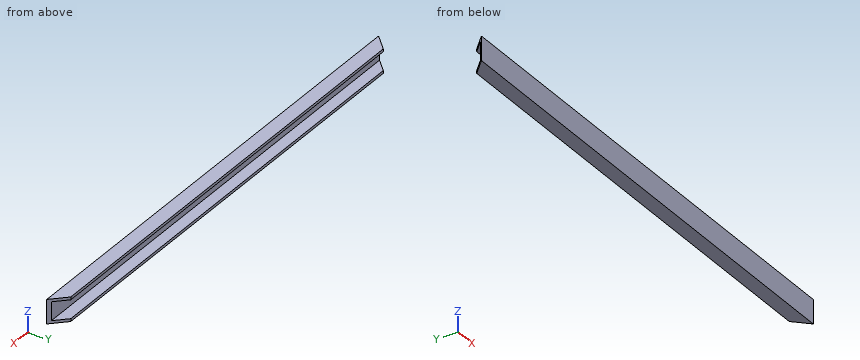
```python
from build123d import *

# Parameters (mm, degrees)
BOSS_EXTRUDE1_DEPTH = 106.2
CUT_EXTRUDE1_DEPTH  = 11.4


with BuildPart() as part:
    # Sketch1 → Boss-Extrude1 (new body, symmetric)
    with BuildSketch(Plane(origin=(0, 0, 0), x_dir=(0, 0, -1), z_dir=(1, 0, 0))):
        Polygon((-4, 5), (-4, 0), (4, 0), (4, 5), (5.2, 5), (5.2, -1.2), (-5.2, -1.2), (-5.2, 5), align=None)
    extrude(amount=BOSS_EXTRUDE1_DEPTH, both=True)

    # Sketch3 → Cut-Extrude1 (cut, through all)
    with BuildSketch(Plane.XY.offset(5.2)):
        Polygon((-106.2, 5), (-106.2, -1.2), (-100, 5), align=None)
        Polygon((106.2, 5), (106.2, -1.2), (100, 5), align=None)
    extrude(amount=-CUT_EXTRUDE1_DEPTH, mode=Mode.SUBTRACT)


solid = part.part
```
Here's how the part is built. I have some questions about the finished solid (model axes, mm). Round coordinates to 2 decimals unless told otherwise and drop trailing zeros. Order: outer loops, then holes, each group sorted by start corner. A loop starts at its lowest first (then second) coordinate and runs counter-clockwise, first axis right, second up. Notation, with made-up numbers: M 84,-21.5 L 110,-21.5 A16 ccw 110,-10.5 Z; hole C 74,80.25 d8. An arc over 180 degrees is marked long. Answer in a Markdown table with one row per item.
Item 1: Imagine slicing it at A-A, the plane y = 2. Write out the boundary of the cut face in (x, z), and give its area (3 significant figures).
A:
| item | result |
|---|---|
| outline | M -103,-5.2 L 103,-5.2 L 103,-4 L -103,-4 Z; M -103,4 L 103,4 L 103,5.2 L -103,5.2 Z |
| area | 494 mm2 |
Item 2: If I drill on L1, parallel to Z at x = 46, y = 0.75; L2, parallel to Y at x = -29, z = 3; L3, parallel to X at y = -0.5, z = 0.75, over which ranges is the centre line in solid material (lowest first)? Write a range as from..to.
A:
| item | result |
|---|---|
| L1 | z = -5.2..-4, 4..5.2 |
| L2 | y = -1.2..0 |
| L3 | x = -105.5..105.5 |
Item 3: Imagine slicing it at B-B, the plane x = -4. Write out the boundary of the cut face in (y, z).
A:
| item | result |
|---|---|
| outline | M -1.2,-5.2 L 5,-5.2 L 5,-4 L 0,-4 L 0,4 L 5,4 L 5,5.2 L -1.2,5.2 Z |
Item 4: Imagine slicing it at C-C, the plane z = 1.75. Write out the boundary of the cut face in (x, y), and give its area (3 significant figures).
A:
| item | result |
|---|---|
| outline | M -106.2,-1.2 L 106.2,-1.2 L 105,0 L -105,0 Z |
| area | 253 mm2 |
